```python
from build123d import *

# Parameters (mm, degrees)
SKETCH2_W           = 138
SKETCH2_H           = 178
BOSS_EXTRUDE1_DEPTH = 5
SKETCH3_W           = 30
SKETCH3_H           = 3
CUT_EXTRUDE1_DEPTH  = 6
SKETCH4_W           = 30
SKETCH4_H           = 3
CUT_EXTRUDE2_DEPTH  = 8
SKETCH6_W           = 3
SKETCH6_H           = 38.70967742
CUT_EXTRUDE3_DEPTH  = 8
SKETCH5_W           = 3
SKETCH5_H           = 40
CUT_EXTRUDE4_DEPTH  = 8
SKETCH8_R           = 1.5
CUT_EXTRUDE5_DEPTH  = 6
SKETCH10_R          = 8
CUT_EXTRUDE8_DEPTH  = 10
SKETCH11_R          = 0.5
CUT_EXTRUDE10_DEPTH = 10


with BuildPart() as part:
    # Sketch2 → Boss-Extrude1 (new body)
    with BuildSketch(Plane.XY):
        Rectangle(SKETCH2_W, SKETCH2_H)
    extrude(amount=BOSS_EXTRUDE1_DEPTH)

    # Sketch3 → Cut-Extrude1 (cut, through all)
    with BuildSketch(Plane.XY.offset(5)):
        with Locations((0, 82.5)):
            Rectangle(SKETCH3_W, SKETCH3_H)
    extrude(amount=-CUT_EXTRUDE1_DEPTH, mode=Mode.SUBTRACT)

    # Sketch4 → Cut-Extrude2 (cut)
    with BuildSketch(Plane.XY.offset(5)):
        with Locations((0, -82.5)):
            Rectangle(SKETCH4_W, SKETCH4_H)
    extrude(amount=-CUT_EXTRUDE2_DEPTH, mode=Mode.SUBTRACT)

    # Sketch6 → Cut-Extrude3 (cut)
    with BuildSketch(Plane.XY.offset(5)):
        with Locations((62.5, 0)):
            Rectangle(SKETCH6_W, SKETCH6_H)
    extrude(amount=-CUT_EXTRUDE3_DEPTH, mode=Mode.SUBTRACT)

    # Sketch5 → Cut-Extrude4 (cut)
    with BuildSketch(Plane.XY.offset(5)):
        with Locations((-62.5, 0)):
            Rectangle(SKETCH5_W, SKETCH5_H)
    extrude(amount=-CUT_EXTRUDE4_DEPTH, mode=Mode.SUBTRACT)

    # Sketch8 → Cut-Extrude5 (cut, through all)
    with BuildSketch(Plane.XY.offset(5)):
        with Locations((54, -74)):
            Circle(SKETCH8_R)
        with Locations((54, 74)):
            Circle(SKETCH8_R)
        with Locations((-54, 74)):
            Circle(SKETCH8_R)
        with Locations((-54, -74)):
            Circle(SKETCH8_R)
    extrude(amount=-CUT_EXTRUDE5_DEPTH, mode=Mode.SUBTRACT)

    # Sketch10 → Cut-Extrude8 (cut)
    with BuildSketch(Plane(origin=(0, 0, 0), x_dir=(-1, 0, 0), z_dir=(0, 0, -1))):
        Circle(SKETCH10_R)
    extrude(amount=-CUT_EXTRUDE8_DEPTH, mode=Mode.SUBTRACT)

    # Sketch11 → Cut-Extrude10 (cut)
    with BuildSketch(Plane(origin=(0, 0, 0), x_dir=(-1, 0, 0), z_dir=(0, 0, -1))):
        with Locations((-3, 45)):
            Circle(SKETCH11_R)
        with Locations((-1.5, 47.598076211)):
            Circle(SKETCH11_R)
        with Locations((1.5, 47.598076211)):
            Circle(SKETCH11_R)
        with Locations((3, 45)):
            Circle(SKETCH11_R)
        with Locations((1.5, 42.401923789)):
            Circle(SKETCH11_R)
        with Locations((-1.5, 42.401923789)):
            Circle(SKETCH11_R)
        with Locations((-6, 45)):
            Circle(SKETCH11_R)
        with Locations((-9, 45)):
            Circle(SKETCH11_R)
        with Locations((-12, 45)):
            Circle(SKETCH11_R)
        with Locations((-15, 45)):
            Circle(SKETCH11_R)
        with Locations((-4.596266659, 48.856725658)):
            Circle(SKETCH11_R)
        with Locations((-1.041889066, 50.908846518)):
            Circle(SKETCH11_R)
        with Locations((3, 50.196152423)):
            Circle(SKETCH11_R)
        with Locations((5.638155725, 47.05212086)):
            Circle(SKETCH11_R)
        with Locations((5.638155725, 42.94787914)):
            Circle(SKETCH11_R)
        with Locations((3, 39.803847577)):
            Circle(SKETCH11_R)
        with Locations((-1.041889066, 39.091153482)):
            Circle(SKETCH11_R)
        with Locations((-4.596266659, 41.143274342)):
            Circle(SKETCH11_R)
        with Locations((-7.794228634, 49.5)):
            Circle(SKETCH11_R)
        with Locations((-4.5, 52.794228634)):
            Circle(SKETCH11_R)
        with Locations((0, 54)):
            Circle(SKETCH11_R)
        with Locations((4.5, 52.794228634)):
            Circle(SKETCH11_R)
        with Locations((7.794228634, 49.5)):
            Circle(SKETCH11_R)
        with Locations((9, 45)):
            Circle(SKETCH11_R)
        with Locations((7.794228634, 40.5)):
            Circle(SKETCH11_R)
        with Locations((4.5, 37.205771366)):
            Circle(SKETCH11_R)
        with Locations((0, 36)):
            Circle(SKETCH11_R)
        with Locations((-4.5, 37.205771366)):
            Circle(SKETCH11_R)
        with Locations((-10.962545492, 49.880839717)):
            Circle(SKETCH11_R)
        with Locations((-8.029567276, 53.917737906)):
            Circle(SKETCH11_R)
        with Locations((-3.708203932, 56.412678196)):
            Circle(SKETCH11_R)
        with Locations((1.254341559, 56.934262744)):
            Circle(SKETCH11_R)
        with Locations((6, 55.392304845)):
            Circle(SKETCH11_R)
        with Locations((9.708203932, 52.053423028)):
            Circle(SKETCH11_R)
        with Locations((11.737771209, 47.49494029)):
            Circle(SKETCH11_R)
        with Locations((11.737771209, 42.50505971)):
            Circle(SKETCH11_R)
        with Locations((9.708203932, 37.946576972)):
            Circle(SKETCH11_R)
        with Locations((6, 34.607695155)):
            Circle(SKETCH11_R)
        with Locations((1.254341559, 33.065737256)):
            Circle(SKETCH11_R)
        with Locations((-3.708203932, 33.587321804)):
            Circle(SKETCH11_R)
        with Locations((-14.095389312, 50.13030215)):
            Circle(SKETCH11_R)
        with Locations((-11.490666647, 54.641814145)):
            Circle(SKETCH11_R)
        with Locations((-7.5, 57.990381057)):
            Circle(SKETCH11_R)
        with Locations((-2.604722665, 59.772116295)):
            Circle(SKETCH11_R)
        with Locations((2.604722665, 59.772116295)):
            Circle(SKETCH11_R)
        with Locations((7.5, 57.990381057)):
            Circle(SKETCH11_R)
        with Locations((11.490666647, 54.641814145)):
            Circle(SKETCH11_R)
        with Locations((14.095389312, 50.13030215)):
            Circle(SKETCH11_R)
        with Locations((15, 45)):
            Circle(SKETCH11_R)
        with Locations((14.095389312, 39.86969785)):
            Circle(SKETCH11_R)
        with Locations((11.490666647, 35.358185855)):
            Circle(SKETCH11_R)
        with Locations((7.5, 32.009618943)):
            Circle(SKETCH11_R)
        with Locations((-7.794228634, 40.5)):
            Circle(SKETCH11_R)
        with Locations((-8.029567276, 36.082262094)):
            Circle(SKETCH11_R)
        with Locations((-10.962545492, 40.119160283)):
            Circle(SKETCH11_R)
        with Locations((2.604722665, 30.227883705)):
            Circle(SKETCH11_R)
        with Locations((-2.604722665, 30.227883705)):
            Circle(SKETCH11_R)
        with Locations((-7.5, 32.009618943)):
            Circle(SKETCH11_R)
        with Locations((-11.490666647, 35.358185855)):
            Circle(SKETCH11_R)
        with Locations((-14.095389312, 39.86969785)):
            Circle(SKETCH11_R)
    extrude(amount=-CUT_EXTRUDE10_DEPTH, mode=Mode.SUBTRACT)


solid = part.part
```
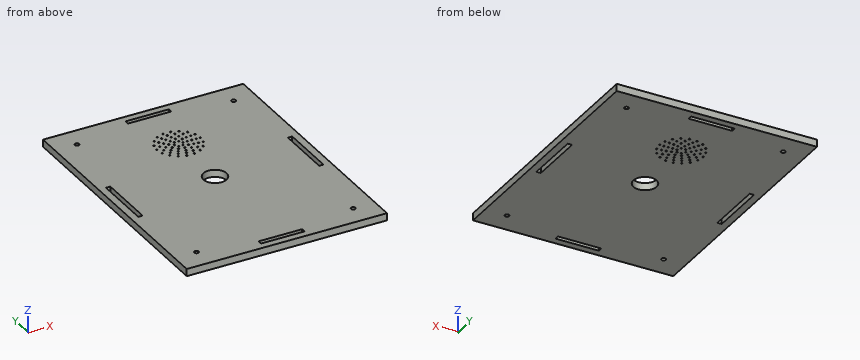
The listing builds one solid part. Answer for the finished solid, in the listing's coordinates (mm). Give positions to 0.01 mm unless a question says otherwise; leave off trailing zeros. Write each loop counter-clockwise with the first axis right and the second up, starting at its lowest first coordinate (ties: lowest second). Pieces come first, ordered by that corner, then holes. Notation, with made-up numbers: M 2,-36 L 17,-36 A11 ccw 17,-29 Z; hole C 1,11.5 d4. An arc over 180 degrees is marked long. Write each question's results on one line, items separated by ' | '.
Q1. Section A-A, the plane y = -10.5 is taken. Write down the section's boundary in (x, z), then the cut area to 3 significant figures.
Output values:
outline: M -69,0 L -64,0 L -64,5 L -69,5 Z; M -61,0 L 61,0 L 61,5 L -61,5 Z; M 64,0 L 69,0 L 69,5 L 64,5 Z | area: 660 mm2
Q2. Consider L1, parallel to Y at x = -14, z = 1.2; L2, parallel to Y at x = -54, z = 2.4; L3, parallel to X at y = -17.5, z = 2.1. Determine where each line is inside the solid, lowest interval first. Write a range as from..to.
Output values:
L1: -89..-84, -81..39.38, 40.36..49.64, 50.62..81, 84..89 | L2: -89..-75.5, -72.5..72.5, 75.5..89 | L3: -69..-64, -61..61, 64..69
Q3. A flat-ended cylindrical pin translates along its axis: P1, Ø14.5, axis at x = 0, y = 0, coming from the -Z side. Find the tip coordinate at first contact, or state that the pin passes through.
Output values:
P1: through
Q4. Section B-B, the plane z = 0.85 is taken. Count the separate pieces of the cut face and the enclosed holes in it, then the cut area to 3 significant figures.
Output values:
separate pieces: 1 | enclosed holes: 69 | area: 23,900 mm2
